Autodesk Inventor part; units mm, degrees
ref_plane "YZ Plane" through (0, 0, 0) normal (1, 0, 0) x (0, 1, 0)
ref_plane "XZ Plane" through (0, 0, 0) normal (0, 1, 0) x (-1, 0, 0)
ref_plane "XY Plane" through (0, 0, 0) normal (0, 0, 1) x (1, 0, 0)
sketch "스케치1" plane through (0, 0, 0) normal (0, 1, 0) x (-1, 0, 0)
  line L0 (0, 0) -> (-270, 0)
  line L1 (-270, 0) -> (-270, -26)
  line L2 (-270, -26) -> (0, -26)
  line L3 (0, -26) -> (0, 0)
  dimension "d0" = 270
  dimension "d1" = 26
extrude "돌출1" add sketch "스케치1" along normal blind 2
sketch "스케치2" plane through (0, 2, 0) normal (0, 1, 0) x (1, 0, 0)
  line L0 (0, 0) -> (270, 0)
  line L1 (270, 0) -> (270, 26)
  line L2 (270, 26) -> (0, 26)
  line L3 (0, 26) -> (0, 0)
  line L4 (1, 26) -> (1, 0)
  line L5 (9.2, 26) -> (9.2, 0)
  line L6 (269, 26) -> (269, 0)
  line L7 (260.8, 26) -> (260.8, 0)
  line L8 (0, 0) -> (270, 0)
  line L9 (270, 26) -> (0, 26)
  line L10 (260.8, 0) -> (269, 0)
  line L11 (260.8, 26) -> (269, 26)
  line L12 (0, 0) -> (40, 0)
  line L13 (40, 0) -> (41, 0)
  line L14 (41, 0) -> (41, 26)
  line L15 (41, 0) -> (49.2, 0)
  line L16 (49.2, 0) -> (49.2, 26)
  line L17 (270, 0) -> (270, 0)
  line L18 (270, 0) -> (229, 0)
  line L19 (229, 0) -> (220.8, 0)
  line L20 (220.8, 0) -> (220.8, 26)
  line L21 (229, 0) -> (229, 26)
  line L22 (229, 26) -> (220.8, 26)
  line L23 (41, 26) -> (49.2, 26)
  line L24 (9.2, 0) -> (1, 0)
  line L25 (9.2, 26) -> (1, 26)
  line L26 (1, 0) -> (1, 26)
  dimension "d19" = 8.2
  dimension "d20" = 1
  dimension "d21" = 8.2
  dimension "d22" = 40
  dimension "d23" = 1
  dimension "d24" = 8.2
  dimension "d26" = 8.2
  dimension "d29" = 41
extrude "돌출3" cut sketch "스케치2" against normal blind 1 contours L4 L2 L5 L0 | L14 L2 L16 L0 | L20 L2 L21 L0 | L7 L2 L6 L0
sketch "스케치5" plane through (0, 0, 0) normal (0, -1, 0) x (1, 0, 0)
  line L0 (0, 0) -> (270, 0)
  line L1 (0, -26) -> (0, 0)
  line L2 (270, -26) -> (0, -26)
  line L3 (270, 0) -> (270, -26)
  line L4 (0, 0) -> (270, 0)
  line L5 (270, -26) -> (0, -26)
  line L6 (127, -26) -> (127, -19)
  line L7 (129, -17) -> (141, -17)
  line L8 (143, -19) -> (143, -26)
  arc A0 (129, -17) -> (127, -19) centre (129, -19) ccw
  arc A1 (143, -19) -> (141, -17) centre (141, -19) ccw
  point P0 (127, -17)
  point P1 (143, -17)
  dimension "d39" = 9
  dimension "d40" = 16
  dimension "d70" = 127
  dimension "d71" = 2
  dimension "d72" = 2
sketch "스케치6" plane through (0, 0, 0) normal (0, -1, 0) x (1, 0, 0)
  line L0 (1, -26) -> (9.2, -26)
  line L1 (1, 0) -> (1, -26)
  line L2 (9.2, 0) -> (1, 0)
  line L3 (9.2, -26) -> (9.2, 0)
  line L4 (49.2, 0) -> (41, 0)
  line L5 (49.2, -26) -> (49.2, 0)
  line L6 (41, -26) -> (49.2, -26)
  line L7 (41, 0) -> (41, -26)
  line L8 (220.8, -26) -> (229, -26)
  line L9 (220.8, 0) -> (220.8, -26)
  line L10 (229, 0) -> (220.8, 0)
  line L11 (229, -26) -> (229, 0)
  line L12 (269, -26) -> (269, 0)
  line L13 (260.8, -26) -> (269, -26)
  line L14 (260.8, 0) -> (260.8, -26)
  line L15 (269, 0) -> (260.8, 0)
  circle A0 centre (5.1, -9) radius 1.5
  circle A1 centre (5.1, -19) radius 1.5
  circle A2 centre (45.1, -9) radius 1.5
  circle A3 centre (45.1, -19) radius 1.5
  circle A4 centre (224.9, -9) radius 1.5
  circle A5 centre (224.9, -19) radius 1.5
  circle A6 centre (264.9, -19) radius 1.5
  circle A7 centre (264.9, -9) radius 1.5
  point P0 (0, 0)
  dimension "d43" = 3
  dimension "d44" = 3
  dimension "d45" = 3
  dimension "d46" = 3
  dimension "d47" = 3
  dimension "d48" = 3
  dimension "d49" = 3
  dimension "d50" = 3
  dimension "d51" = 4.1
  dimension "d52" = 4.1
  dimension "d53" = 4.1
  dimension "d54" = 4.1
  dimension "d55" = 4.1
  dimension "d56" = 4.1
  dimension "d57" = 4.1
  dimension "d58" = 4.1
  dimension "d59" = 9
  dimension "d60" = 7
  dimension "d61" = 7
  dimension "d62" = 9
  dimension "d63" = 9
  dimension "d64" = 7
  dimension "d65" = 7
  dimension "d66" = 9
extrude "돌출6" cut sketch "스케치6" against normal blind 10 contours A0 | A1 | A2 | A3 | A4 | A5 | A6 | A7
extrude "돌출7" cut sketch "스케치5" against normal blind 2 contours L6 A0 L7 A1 L8 L2
sketch "스케치7" plane through (0, 2, 0) normal (0, 1, 0) x (1, 0, 0)
  line L0 (127, 19) -> (127, 26)
  line L1 (127, 26) -> (49.2, 26)
  line L2 (49.2, 26) -> (49.2, 0)
  line L3 (49.2, 0) -> (220.8, 0)
  line L4 (220.8, 0) -> (220.8, 26)
  line L5 (220.8, 26) -> (143, 26)
  line L6 (143, 26) -> (143, 19)
  arc A0 (141, 17) -> (143, 19) centre (141, 19) ccw
  line L7 (141, 17) -> (129, 17)
  arc A1 (127, 19) -> (129, 17) centre (129, 19) ccw
  line L8 (49.2, 0) -> (220.8, 0)
  line L9 (270, 26) -> (143, 26)
  line L10 (172, 0) -> (163.8, 0)
  line L11 (163.8, 0) -> (163.8, 26)
  line L12 (163.8, 26) -> (172, 26)
  line L13 (172, 26) -> (172, 0)
  line L14 (127, 26) -> (49.2, 26)
  line L15 (106.2, 0) -> (98, 0)
  line L16 (98, 0) -> (98, 26)
  line L17 (98, 26) -> (106.2, 26)
  line L18 (106.2, 26) -> (106.2, 0)
  line L19 (270, 0) -> (270, 26)
  line L20 (0, 26) -> (0, 0)
  dimension "d75" = 8.2
  dimension "d76" = 8.2
  dimension "d77" = 98
  dimension "d78" = 98
extrude "돌출8" cut sketch "스케치7" against normal blind 1 contours L18 L3 L16 L1 | L11 L5 L13 L3
sketch "스케치8" plane through (0, 1, 0) normal (0, 1, 0) x (1, 0, 0)
  circle A0 centre (167.9, 19) radius 1.5
  circle A1 centre (167.9, 9) radius 1.5
  circle A2 centre (102.1, 9) radius 1.5
  circle A3 centre (102.1, 19) radius 1.5
  line L0 (163.8, 26) -> (172, 26)
  line L1 (172, 26) -> (172, 0)
  line L2 (163.8, 0) -> (163.8, 26)
  line L3 (106.2, 26) -> (106.2, 0)
  line L4 (98, 0) -> (98, 26)
  line L5 (98, 26) -> (106.2, 26)
  point P0 (0, 0)
  dimension "d81" = 3
  dimension "d82" = 3
  dimension "d83" = 3
  dimension "d84" = 3
  dimension "d85" = 7
  dimension "d86" = 4.1
  dimension "d87" = 4.1
  dimension "d88" = 10
  dimension "d89" = 4.1
  dimension "d90" = 4.1
  dimension "d91" = 7
  dimension "d92" = 10
extrude "돌출9" cut sketch "스케치8" against normal blind 1
sketch "스케치9" plane through (0, 2, 0) normal (0, 1, 0) x (1, 0, 0)
  line L0 (230, 0) -> (230, 25)
  line L1 (40, 25) -> (40, 0)
  line L2 (270, 0) -> (270, 26)
  line L3 (230, 0) -> (270, 0)
  line L4 (270, 0) -> (270, 26)
  line L5 (270, 26) -> (230, 26)
  line L6 (230, 26) -> (230, 0)
  line L7 (40, 0) -> (0, 0)
  line L8 (0, 0) -> (0, 26)
  line L9 (0, 26) -> (40, 26)
  line L10 (40, 26) -> (40, 0)
extrude "돌출10" cut sketch "스케치9" against normal blind 10
properties part number "앞뒷판_중간" material "알루미늄 6061"
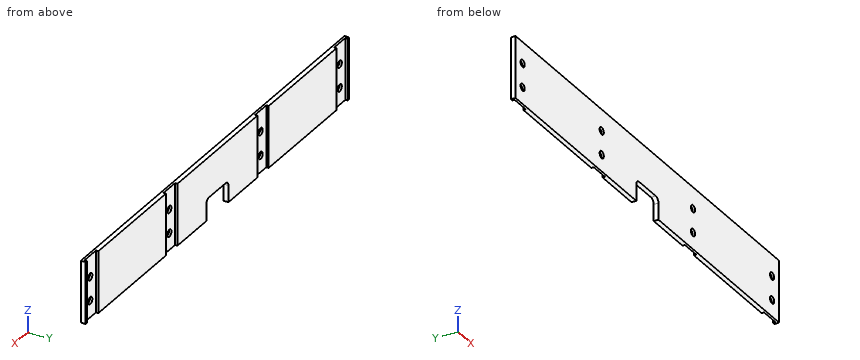
Source: CAD feature listing. Evaluate the final solid. Frame: model axes, mm. Coordinates: 2 decimals unless noted, no trailing zeros. Loops run counter-clockwise (first coordinate to the right, second up) from the corner with the lowest first, then second, coordinate; pieces in that order, holes last. Notation, with made-up numbers: (22.5, -9) - (45.5, -9) arc R15 ccw to (45.5, 1) - close; hole circle Ø8 at (1.25, 64). An arc over 180 degrees is marked (long way). One line per question, with ' | ' between items.
1) First-contact query: P1, Ø6.5, axis at x = 224.5, z = -13, coming from the +Y side; P2, Ø1.8, axis at x = 224.9, z = -9, coming from the -Y side. Flat tips, straight axial feed; report the tip coordinate or a pass-through.
Report:
P1: stops at y = 1 | P2: passes through
2) Line query: line 1 along X through (y, z) = (1.3, -7.25); line 2 along X through (y, z) = (0.3, -20); line 3 along Y through (x, z) = (169.5, -12). Output: solid intervals per line, ascending.
Report:
line 1: x = 40 to 41, 49.2 to 98, 106.2 to 163.8, 172 to 220.8, 229 to 230 | line 2: x = 40 to 43.98, 46.22 to 100.98, 103.22 to 127, 143 to 166.78, 169.02 to 223.78, 226.02 to 230 | line 3: y = 0 to 1
3) Section A-A, the plane z = -22.5. Return loops of the section in (x, y).
Report:
outline: (40, 0) - (127, 0) - (127, 2) - (106.2, 2) - (106.2, 1) - (98, 1) - (98, 2) - (49.2, 2) - (49.2, 1) - (41, 1) - (41, 2) - (40, 2) - close; (143, 0) - (230, 0) - (230, 2) - (229, 2) - (229, 1) - (220.8, 1) - (220.8, 2) - (172, 2) - (172, 1) - (163.8, 1) - (163.8, 2) - (143, 2) - close
4) Section B-B, the plane y = 1.6. Return loops of the section in (x, z).
Report:
outline: (40, -26) - (41, -26) - (41, 0) - (40, 0) - close; (49.2, -26) - (98, -26) - (98, 0) - (49.2, 0) - close; (106.2, -26) - (127, -26) - (127, -19) arc R2 cw to (129, -17) - (141, -17) arc R2 cw to (143, -19) - (143, -26) - (163.8, -26) - (163.8, 0) - (106.2, 0) - close; (172, -26) - (220.8, -26) - (220.8, 0) - (172, 0) - close; (229, -26) - (230, -26) - (230, 0) - (229, 0) - close
